from build123d import *

# Parameters (mm, degrees)
F0_W     = 4
F0_H     = 30
F1_DEPTH = 200


with BuildPart() as f1:
    # F0 (on Front) → F1 (new body)
    with BuildSketch(Plane.XZ):
        with Locations((0, 18)):
            Rectangle(F0_W, F0_H)
        Polygon((-2, 3), (-20, 3), (-20, 0), (20, 0), (20, 3), (2, 3), align=None)
    extrude(amount=F1_DEPTH)


solid = f1.part
Model file for the job. Use its own axes, mm. A direction names the side the tool comes from. Give positions to 0.01 mm unless a question says otherwise; leave off trailing zeros. Write each loop counter-clockwise with the first axis right and the second up, starting at its lowest first coordinate (ties: lowest second). Pieces come first, ordered by that corner, then holes. Notation, with made-up numbers: M 63.5,74 L 92.5,74 A18 ccw 92.5,81 Z; hole C -8,-5.75 d5. An arc over 180 degrees is marked long. One line per item, written item: value. Start each with the question number.
Q1. 3-axis set-ups, long thin cutter, end or side, ignore diameter. For faces 1 (the flat face through (-11, -99, 3)), 2 (the flat face through (0, -99, 0)), 3 (the flat face through (2, -99, 18)): which of +Z, -Z, +X, -X, +Y, -Y reach the whole face in a straight line?
Q2. Saw through at C-C, the plane z = 24.5. Write the cut outline in (x, y).
Q3. Saw through at A-A, the plane y = -83.5. Write the cut outline in (x, z), plus the area to 3 significant figures.
Q4. Probe probe 1 along X at (y, z) = (-163, 9.5); probe 2 along Z at (x, y) = (-15, -131). List the from-to ranges inside material, lowest first. Write a range as [from, to].
Q5. Drop flat-ended pins along their axis: pin 1 Ø14.5 at (x, y) = (-12, -82) entering from +Z; pin 2 Ø1.5 at (y, z) = (-154.5, 22.5) entering from -X; pin 3 Ø8 at (y, z) = (-96, 27) entering from +X. Give the stop position or say it passes through.
Q6. Saw through at B-B, the plane x = 9. Write the cut outline in (y, z), plus the area to 3 significant figures.
Output values:
1. face 1: +Z, -X, +Y, -Y
1. face 2: -Z, +X, -X, +Y, -Y
1. face 3: +Z, +X, +Y, -Y
2. outline: M -2,-200 L 2,-200 L 2,0 L -2,0 Z
3. outline: M -20,0 L 20,0 L 20,3 L 2,3 L 2,33 L -2,33 L -2,3 L -20,3 Z
3. area: 240 mm²
4. probe 1: x = [-2, 2]
4. probe 2: z = [0, 3]
5. pin 1: stops at z = 3
5. pin 2: stops at x = -2
5. pin 3: stops at x = 2
6. outline: M -200,0 L 0,0 L 0,3 L -200,3 Z
6. area: 600 mm²
